Geometry: final body of the model. Coordinates: model frame, mm. Coordinates: 2 decimals unless noted, no trailing zeros. Order: outer loops, then holes, each group sorted by start corner. A loop starts at its lowest first (then second) coordinate and runs counter-clockwise, first axis right, second up. Notation, with made-up numbers: (71.5, -37.5) - (88.5, -37.5) arc R34 ccw to (88.5, -5.5) - close; hole circle Ø10 at (-10, 75.25). An arc over 180 degrees is marked (long way). Use a Markdown table: item, result. Add a question column.
Autodesk Inventor part; units mm, degrees
ref_plane "YZ Plane" through (0, 0, 0) normal (1, 0, 0) x (0, 1, 0)
ref_plane "XZ Plane" through (0, 0, 0) normal (0, 1, 0) x (-1, 0, 0)
ref_plane "XY Plane" through (0, 0, 0) normal (0, 0, 1) x (1, 0, 0)
sketch "Sketch1" plane through (0, 0, 0) normal (0, 0, 1) x (1, 0, 0)
  circle A0 centre (0, 0) radius 22.5
  circle A1 centre (140, 0) radius 22.5
  arc A2 (6.3, 21.6) -> (133.7, 21.6) centre (70, 240) ccw
  line L0 (162.5, 0) -> (-22.5, 0) construction
  arc A3 (133.7, -21.6) -> (6.3, -21.6) centre (70, -240) ccw
  circle A4 centre (0, 0) radius 5
  circle A5 centre (140, 0) radius 5
  point P0 (70, 12.5)
  point P1 (6.3, -21.6)
  point P2 (133.7, -21.6)
  dimension "d0" = 45
  dimension "d1" = 140
  dimension "d2" = 12.5
  dimension "d3" = 10
  dimension "d4" = 10
extrude "Extrusion1" add sketch "Sketch1" along normal mid plane 2
properties part number "stelscharnier bovenkant" material "Stainless Steel"
1) Section D-D (z = 0.1). Return loops of the section in (x, y).
2) Section B-B (x = 140). Return loops of the section in (y, z), then the cut area to 3 significant figures.
3) Section C-C (y = 19.5). Return loops of the section in (x, z), then the cut area to 3 significant figures.
4) Pin query (flat end, axial travel): pin 1 (13 mm diameter, centred on x = 0, y = 0, fed in from +Z); pin 2 (1 mm diameter, centred on x = 56.5, z = 0, fed in from -Y). Return the tip coordinate at first contact, or that it passes through.
5) Ray query, line 1 along Y through (x, z) = (0, 0.25); line 2 along Y through (x, z) = (143.5, -0.2); line 3 along X through (y, z) = (2, 0.4). Return the intervals inside material, ascending.
6) Draft query along Y for faces 1 (the face through (136, 3, 0)), 2 (the face through (70.9, 12.5, 0)), 3 (the face through (162.492, 0.584, -0.014)). Return one class per face: pulls with the +Y half, pulls with the -Y half, needs draft (parallel to the pull), parting line crosses it, or undercut.
7) Section A-A (y = 0). Return loops of the section in (x, z), then the cut area to 3 significant figures.
Values follow:
| question | item | result |
|---|---|---|
| 1 | outline | (6.3, -21.6) arc R227.5 cw to (133.7, -21.6) arc R22.5 ccw (long way) to (133.7, 21.6) arc R227.5 cw to (6.3, 21.6) arc R22.5 ccw (long way) to start; hole circle Ø10 at (0, 0); hole circle Ø10 at (140, 0) |
| 2 | outline | (-22.5, -1) - (-5, -1) - (-5, 1) - (-22.5, 1) - close; (5, -1) - (22.5, -1) - (22.5, 1) - (5, 1) - close |
| 2 | area | 70.0 mm² |
| 3 | outline | (-11.22, -1) - (14, -1) - (14, 1) - (-11.22, 1) - close; (126, -1) - (151.22, -1) - (151.22, 1) - (126, 1) - close |
| 3 | area | 101 mm² |
| 4 | pin 1 | stops at z = 1 |
| 4 | pin 2 | stops at y = -12.93 |
| 5 | line 1 | y = -22.5 to -5, 5 to 22.5 |
| 5 | line 2 | y = -22.23 to -3.57, 3.57 to 22.23 |
| 5 | line 3 | x = -22.41 to -4.58, 4.58 to 135.42, 144.58 to 162.41 |
| 6 | face 1 | undercut |
| 6 | face 2 | pulls with the +Y half |
| 6 | face 3 | parting line crosses it |
| 7 | outline | (-22.5, -1) - (-5, -1) - (-5, 1) - (-22.5, 1) - close; (5, -1) - (135, -1) - (135, 1) - (5, 1) - close; (145, -1) - (162.5, -1) - (162.5, 1) - (145, 1) - close |
| 7 | area | 330 mm² |
